Can you work these out from the model? Positions are in its coordinate system, mm. Face numbers are marked on the shaded views. A direction names the side the tool comes from. Give positions to 0.01 mm unless a question says otherwise; leave off trailing zeros. Loops run counter-clockwise (first coordinate to the right, second up) from the corner with the lowest first, then second, coordinate; pieces in that order, holes last. Notation, with made-up numbers: (-2.5, 13.25) - (55.5, 13.25) arc R11 ccw to (55.5, 31.25) - close; hole circle Ø4 at (13.25, -33). An arc over 180 degrees is marked (long way). Answer in a Markdown table with one row per item.
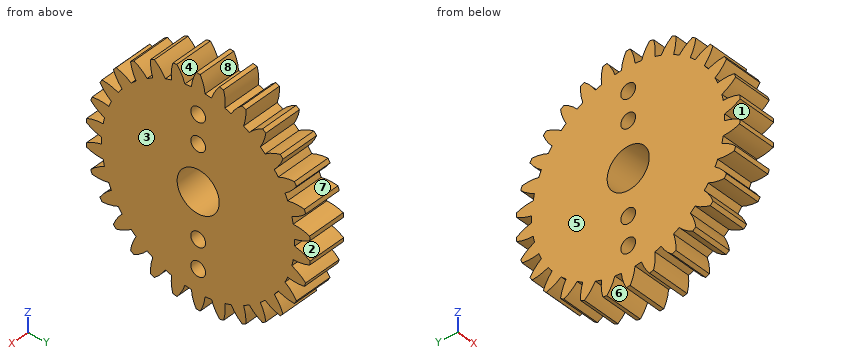
from build123d import *

# Parameters (mm, degrees)
BASPROSKE_W         = 5.5
BASPROSKE_H         = 16
TOOTHCUT_DEPTH      = 24.286262044
TEETHCUTS_COUNT     = 30
TEETHCUTS_ANGLE     = 348
BORSKE_R            = 0.5
BORE_DEPTH          = 50.0000508
SKETCH_1_R          = 3
SKETCH_1_R_2        = 1.05
CUT_EXTRUDE_1_DEPTH = 24.245268194


with BuildPart() as part:
    # BasProSke → Base-Revolve (revolve)
    with BuildSketch(Plane(origin=(0, 0, 0), x_dir=(1, 0, 0), z_dir=(0, 1, 0)), mode=Mode.PRIVATE) as base_revolve_sk:
        with Locations((2.75, 8)):
            Rectangle(BASPROSKE_W, BASPROSKE_H)
    revolve(base_revolve_sk.sketch.rotate(Axis((-10, 0, 0), (1, 0, 0)), 180), axis=Axis((-10, 0, 0), (1, 0, 0)))

    # TooCutSke → ToothCut (cut, through all)
    with BuildSketch(Plane(origin=(0, 0, 0), x_dir=(0, 0, -1), z_dir=(1, 0, 0))):
        with BuildLine():
            ThreePointArc((0.466400716, 13.741086979), (0, 13.749), (-0.466400716, 13.741086979))
            ThreePointArc((-0.466400716, 13.741086979), (-0.819142092, 14.899954875), (-1.3974676, 15.964351834))
            ThreePointArc((-1.3974676, 15.964351834), (0, 16.0254), (1.3974676, 15.964351834))
            ThreePointArc((1.3974676, 15.964351834), (0.819142092, 14.899954875), (0.466400716, 13.741086979))
        make_face()
    toothcut = extrude(amount=TOOTHCUT_DEPTH, mode=Mode.SUBTRACT)

    # TeethCuts: ToothCut ×30 about axis
    teethcuts_axis = Axis((-10, 0, 0), (1, 0, 0))
    for i in range(1, TEETHCUTS_COUNT):
        add(toothcut.rotate(teethcuts_axis, i * TEETHCUTS_ANGLE / (TEETHCUTS_COUNT - 1)), mode=Mode.SUBTRACT)

    # BorSke → Bore (cut, symmetric)
    with BuildSketch(Plane(origin=(0, 0, 0), x_dir=(0, 0, -1), z_dir=(1, 0, 0))):
        with Locations(Location((0, 0, 0), (0, 0, 180))):
            Circle(BORSKE_R)
    extrude(amount=BORE_DEPTH, both=True, mode=Mode.SUBTRACT)

    # ｽｹｯﾁ1 → ｶｯﾄ - 押し出し1 (cut, through all)
    with BuildSketch(Plane(origin=(5.5, 0, 0), x_dir=(0, 0, -1), z_dir=(1, 0, 0))):
        Circle(SKETCH_1_R)
        with Locations((6.45, 0)):
            Circle(SKETCH_1_R_2)
        with Locations((10.45, 0)):
            Circle(SKETCH_1_R_2)
        with Locations((-6.45, 0)):
            Circle(SKETCH_1_R_2)
        with Locations((-10.45, 0)):
            Circle(SKETCH_1_R_2)
    extrude(amount=-CUT_EXTRUDE_1_DEPTH, mode=Mode.SUBTRACT)


solid = part.part
Q1. On a 3-axis mill with a long thin cutter (end or side, diameter ignored), from which of +Z, -Z, +X, -X, +Y, -Y can I reach the whole of each face in a straight line? I mean the marked faces 5, 6, 7 and 8. Say none if no direction works.
Checked values:
| item | result |
|---|---|
| face 5 | +Z, -Z, -X, +Y, -Y |
| face 6 | -Z, +X, -X |
| face 7 | +X, -X |
| face 8 | +Z, +X, -X |
Q2. If I drill on line 1 (Y direction, x = 4.15, z = 0); line 2 (Z direction, x = 4.15, y = 13); line 3 (Z direction, x = 1.5, y = 11), over which ranges is the centre line in solid material (lowest first)? Write a range as [from, to].
Checked values:
| item | result |
|---|---|
| line 1 | y = [-13.75, -3], [3, 13.75] |
| line 2 | z = [-8.19, -6.53], [-5.22, 5.22], [6.53, 8.19] |
| line 3 | z = [-10.7, -8.63], [-8.25, 8.25], [8.63, 10.7] |
Q3. Imagine slicing it at C-C, the plane z = -6.45. Write out the boundary of the cut face in (x, y), and give its area (3 significant figures).
Checked values:
| item | result |
|---|---|
| outline | (0, -12.91) - (5.5, -12.91) - (5.5, -1.05) - (0, -1.05) - close; (0, 1.05) - (5.5, 1.05) - (5.5, 12.91) - (0, 12.91) - close |
| area | 130 mm² |
Q4. If we mould it in two halves opening along Y, with no side actions, what happens to the marked faces 1, 2, 3 and 4? For each: released by +Y, released by -Y, zero draft, split by the parting line, or undercut.
Checked values:
| item | result |
|---|---|
| face 1 | released by -Y |
| face 2 | released by +Y |
| face 3 | zero draft |
| face 4 | undercut |
Q5. Imagine slicing it at A-A, the plane z = 0. Write out the boundary of the cut face in (x, y), and give its area (3 significant figures).
Checked values:
| item | result |
|---|---|
| outline | (0, -13.75) - (5.5, -13.75) - (5.5, -3) - (0, -3) - close; (0, 3) - (5.5, 3) - (5.5, 13.75) - (0, 13.75) - close |
| area | 118 mm² |
Q6. For pin 1 (4 mm diameter, centred on y = -4.5, z = -11, fed in from -X), with a flat end and sliding along its axis, tell me the tip position at first contact or that it passes through.
Checked values:
| item | result |
|---|---|
| pin 1 | stops at x = 0 |
Q7. Imagine slicing it at B-B, the plane x = 2. Count the separate pieces of the cut face and the enclosed holes in it, and give its area (3 significant figures).
Checked values:
| item | result |
|---|---|
| separate pieces | 1 |
| enclosed holes | 5 |
| area | 648 mm² |
